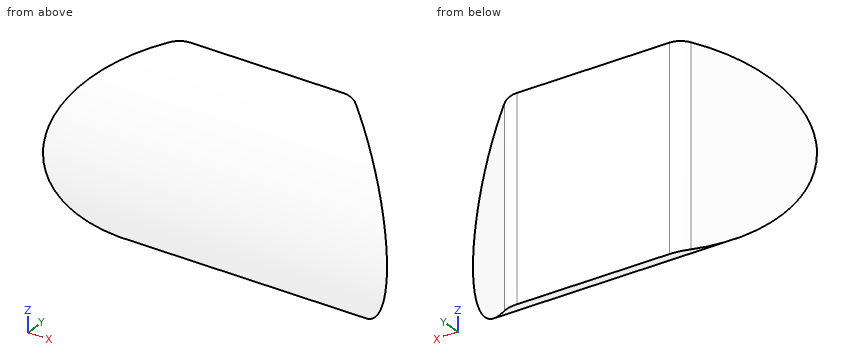
from build123d import *

# Parameters (mm, degrees)
BOSS_EXTRUDE1_DEPTH = 127
CUT_EXTRUDE3_DEPTH  = 166.314783368
FILLET3_R           = 19.05


with BuildPart() as part:
    # Sketch1 → Boss-Extrude1 (new, symmetric)
    with BuildSketch(Plane(origin=(0, 0, 0), x_dir=(0, 0, -1), z_dir=(1, 0, 0))):
        with BuildLine():
            Line((-73.440708058, -20.32), (73.440708058, -20.32))
            ThreePointArc((73.440708058, -20.32), (0, -76.2), (-73.440708058, -20.32))
        make_face()
    extrude(amount=BOSS_EXTRUDE1_DEPTH, both=True)

    # Sketch7 → Cut-Extrude3 (cut, symmetric)
    with BuildSketch(Plane.XY):
        Polygon((-63.5, -20.32), (-127, -20.32), (-127, -76.2), align=None)
    cut_extrude3 = extrude(amount=CUT_EXTRUDE3_DEPTH, both=True, mode=Mode.SUBTRACT)

    # Mirror4: Cut-Extrude3 across plane
    add(cut_extrude3.mirror(Plane(origin=(0, 0, 0), x_dir=(0, 0, 1), z_dir=(1, 0, 0))), mode=Mode.SUBTRACT)

    # Fillet3
    fillet3_edges = [part.edges().sort_by_distance(p)[0] for p in [
        (63.5, -20.32, 0),
        (-63.5, -20.32, 0),
    ]]
    fillet(fillet3_edges, radius=FILLET3_R)


with BuildPart() as body_2:
    # Split1: the piece on the far side of the plane
    add(part.part)
    split(bisect_by=Plane(origin=(0, 0, 0), x_dir=(0, 0, 1), z_dir=(1, 0, 0)), keep=Keep.BOTTOM)


with BuildPart() as part_1:
    add(part.part)

    # Split1
    split(bisect_by=Plane(origin=(0, 0, 0), x_dir=(0, 0, 1), z_dir=(1, 0, 0)), keep=Keep.TOP)


with BuildPart() as body_2_1:
    add(body_2.part)

    # Combine1: union part
    add(part_1.part)


solid = body_2_1.part
Could you check a few things on this model? Use its own coordinates, in mm. Coordinates: 2 decimals unless noted, no trailing zeros. Order: outer loops, then holes, each group sorted by start corner. A loop starts at its lowest first (then second) coordinate and runs counter-clockwise, first axis right, second up. Notation, with made-up numbers: (67.25, 87.25) - (76.25, 87.25) arc R25 cw to (76.25, 115.25) - close; hole circle Ø5 at (-23.5, 63.5). An arc over 180 degrees is marked (long way). Answer in a Markdown table with one row per item. Add a question column.
(1) If we section it at D-D, the plane z = 40: Please give me the cut outline in (x, y).
(2) Will these pins go through, and if not, where does the flat tip stop? pin 1 (1.5 mm diameter, centred on x = 59, z = -24.5, fed in from +Y); pin 2 (1.5 mm diameter, centred on y = -53, z = -3.5, fed in from +X); pin 3 (10 mm diameter, centred on x = 81.5, y = -50.5, fed in from -Z); pin 4 (10 mm diameter, centred on y = -70.5, z = 44, fed in from +X).
(3) If we section it at B-B, the plane y = -52: Please give me the cut outline in (x, z).
(4) If we section it at C-C, the plane x = 5: Please give me the cut outline in (y, z).
(5) I need wall thicknesses on L1, parallel to Y at x = -65.5, z = -49; L2, parallel to Z at x = 49, y = -48.5; L3, parallel to Y at x = 104, z = 23. Which ranges of each line are inside material? Lowest first, please.
(6) If we section it at A-A, the plane z = -58.5: Please give me the cut outline in (x, y), then the cut area to 3 significant figures.
Results are:
| question | item | result |
|---|---|---|
| 1 | outline | (-114.11, -64.86) - (114.11, -64.86) - (68.9, -25.07) arc R19.05 ccw to (56.31, -20.32) - (-56.31, -20.32) arc R19.05 ccw to (-68.9, -25.07) - close |
| 2 | pin 1 | stops at y = -20.42 |
| 2 | pin 2 | stops at x = 101.49 |
| 2 | pin 3 | stops at z = -61.12 |
| 2 | pin 4 | passes through |
| 3 | outline | (-99.5, -55.7) - (99.5, -55.7) - (99.5, 55.7) - (-99.5, 55.7) - close |
| 4 | outline | (-20.32, -73.44) - (-20.32, 73.44) arc R76.2 ccw to start |
| 5 | L1 | y = -58.36 to -22.68 |
| 5 | L2 | z = -58.77 to 58.77 |
| 5 | L3 | y = -72.65 to -55.96 |
| 6 | outline | (-95.9, -48.83) - (95.9, -48.83) - (68.9, -25.07) arc R19.05 ccw to (56.31, -20.32) - (-56.31, -20.32) arc R19.05 ccw to (-68.9, -25.07) - close |
| 6 | area | 4,530 mm2 |
